Work out the finished part from the listing and answer in its coordinate system (mm). Coordinates: 2 decimals unless noted, no trailing zeros. Order: outer loops, then holes, each group sorted by start corner. A loop starts at its lowest first (then second) coordinate and runs counter-clockwise, first axis right, second up. Notation, with made-up numbers: M 0,24 L 20,24 A29 cw 20,60 Z; hole C -28,36 d9. An arc over 180 degrees is marked long. Use a Markdown table: item, result.
from build123d import *

# Parameters (mm, degrees)
SKETCH2_R           = 20
BOSS_EXTRUDE1_DEPTH = 400
SKETCH3_W           = 8.124111934
SKETCH3_H           = 23.526074142
CUT_EXTRUDE1_DEPTH  = 24
SKETCH5_W           = 21.791522519
SKETCH5_H           = 7.386956786
CUT_EXTRUDE2_DEPTH  = 17
SKETCH5_2_W         = 21.791522519
SKETCH5_2_H         = 7.386956786
CUT_EXTRUDE3_DEPTH  = 11


with BuildPart() as part:
    # Sketch2 → Boss-Extrude1 (new body)
    with BuildSketch(Plane(origin=(0, 0, 0), x_dir=(0, 0, -1), z_dir=(1, 0, 0))):
        Circle(SKETCH2_R)
    extrude(amount=BOSS_EXTRUDE1_DEPTH)

    # Sketch3 → Cut-Extrude1 (cut)
    with BuildSketch(Plane(origin=(0, 20, 0), x_dir=(1, 0, 0), z_dir=(0, 1, 0))):
        with Locations((14.062055967, -0.008909978)):
            Rectangle(SKETCH3_W, SKETCH3_H)
    extrude(amount=-CUT_EXTRUDE1_DEPTH, mode=Mode.SUBTRACT)

    # Sketch5 → Cut-Extrude2 (cut)
    with BuildSketch(Plane.ZY.offset(-18.124111934)):
        with Locations((-0.659549714, -0.342965851)):
            Rectangle(SKETCH5_W, SKETCH5_H)
    extrude(amount=-CUT_EXTRUDE2_DEPTH, mode=Mode.SUBTRACT)

    # Sketch5<2> → Cut-Extrude3 (cut)
    with BuildSketch(Plane.ZY.offset(-18.124111934)):
        with Locations((-0.659549714, -0.342965851)):
            Rectangle(SKETCH5_2_W, SKETCH5_2_H)
    extrude(amount=CUT_EXTRUDE3_DEPTH, mode=Mode.SUBTRACT)


solid = part.part
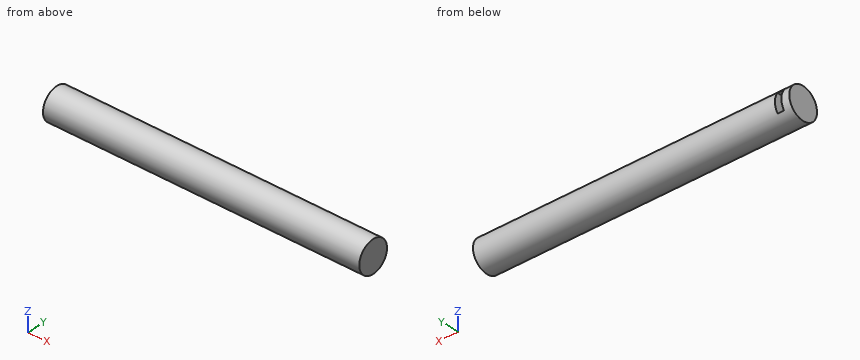
1. Find the intervals of material crossed by probe 1 along X at (y, z) = (-2, -3.5); probe 2 along X at (y, z) = (14, 1.5); probe 3 along Y at (x, z) = (313.5, 0.5), in increasing order.
Answers below:
| item | result |
|---|---|
| probe 1 | 0 to 7.12, 35.12 to 400 |
| probe 2 | 0 to 10, 18.12 to 400 |
| probe 3 | -19.99 to 19.99 |
2. Section B-B on z = 0 is taken. Determine the outline of the cut face in (x, y), then the cut area to 3 significant figures.
Answers below:
| item | result |
|---|---|
| outline | M 0,-20 L 400,-20 L 400,20 L 18.12,20 L 18.12,3.35 L 35.12,3.35 L 35.12,-4.04 L 7.12,-4.04 L 7.12,3.35 L 10,3.35 L 10,20 L 0,20 Z |
| area | 15,700 mm² |
3. Section C-C on x = 343 is taken. Determine the outline of the cut face in (y, z).
Answers below:
| item | result |
|---|---|
| outline | C 0,0 d40 |
4. Flat-ended cylindrical pins translate along their axes: P1, Ø0.9, axis at x = 9, z = 1, coming from the -Y side; P2, Ø4, axis at x = 14, y = 5.5, coming from the +Z side; P3, Ø6, axis at x = 118.5, y = 5, coming from the -Z side. Find the tip coordinate at first contact, or state that the pin passes through.
Answers below:
| item | result |
|---|---|
| P1 | y = -19.99 |
| P2 | z = 19.69 |
| P3 | z = -19.9 |
5. Section A-A on y = 0 is taken. Determine the outline of the cut face in (x, z).
Answers below:
| item | result |
|---|---|
| outline | M 0,-20 L 400,-20 L 400,20 L 0,20 Z; hole M 7.12,-11.56 L 10,-11.56 L 10,-11.75 L 18.12,-11.75 L 18.12,-11.56 L 35.12,-11.56 L 35.12,10.24 L 18.12,10.24 L 18.12,11.77 L 10,11.77 L 10,10.24 L 7.12,10.24 Z |
6. Section D-D on y = -15 is taken. Determine the outline of the cut face in (x, z), then the cut area to 3 significant figures.
Answers below:
| item | result |
|---|---|
| outline | M 0,-13.23 L 400,-13.23 L 400,13.23 L 0,13.23 Z |
| area | 10,600 mm² |
